from build123d import *

# Parameters (mm, degrees)
BLANKSKE_W           = 127
BLANKSKE_H           = 43.18
BLANK_DEPTH          = 25.4
TOOTHCUTSIM_DEPTH    = 137.523523248
TEETHCUTS_COUNT      = 9
TEETHCUTS_PITCH      = 15.959290662
BOSS_EXTRUDE1_DEPTH  = 25.4
MIRROR1_COPY_1_DEPTH = 137.523523248
MIRROR1_COPY_2_DEPTH = 137.523523248
MIRROR1_COPY_3_DEPTH = 137.523523248
MIRROR1_COPY_4_DEPTH = 137.523523248
MIRROR1_COPY_5_DEPTH = 137.523523248
MIRROR1_COPY_6_DEPTH = 137.523523248
MIRROR1_COPY_7_DEPTH = 137.523523248
MIRROR1_COPY_8_DEPTH = 137.523523248
CUT_EXTRUDE1_DEPTH   = 232.151804304
SKETCH5_W            = 249.809436719
SKETCH5_H            = 19.05
CUT_EXTRUDE2_DEPTH   = 232.151804304
BOSS_EXTRUDE2_DEPTH  = 6.35


with BuildPart() as part:
    # BlankSke → Blank (new body)
    with BuildSketch(Plane.XY):
        with Locations((63.5, 21.59)):
            Rectangle(BLANKSKE_W, BLANKSKE_H)
    blank = extrude(amount=-BLANK_DEPTH)

    # TooCutSkeSim → ToothCutSim (cut, through all)
    with BuildSketch(Plane.XY):
        Polygon((2.250111678, 31.75), (-2.250111678, 31.75), (-6.4195363, 43.2054), (6.4195363, 43.2054), align=None)
    toothcutsim = extrude(amount=-TOOTHCUTSIM_DEPTH, mode=Mode.SUBTRACT)

    # TeethCuts: ToothCutSim ×9
    with Locations(*[(i * TEETHCUTS_PITCH, 0, 0) for i in range(1, TEETHCUTS_COUNT)]):
        add(toothcutsim, mode=Mode.SUBTRACT)

    # Sketch3 → Boss-Extrude1 (add)
    with BuildSketch(Plane(origin=(0, 0, -25.4), x_dir=(-1, 0, 0), z_dir=(0, 0, -1))):
        with BuildLine():
            Line((-127.960169835, 127), (-5.150733116, 127))
            ThreePointArc((-5.150733116, 127), (58.349266884, 63.5), (-5.150733116, 0))
            Line((-5.150733116, 0), (-127.960169835, 0))
            ThreePointArc((-127.960169835, 0), (-191.460169835, 63.5), (-127.960169835, 127))
        make_face()
        with BuildLine():
            Line((-127.960169835, 95.25), (-5.150733116, 95.25))
            ThreePointArc((-5.150733116, 95.25), (26.599266884, 63.5), (-5.150733116, 31.75))
            Line((-5.150733116, 31.75), (-127.960169835, 31.75))
            ThreePointArc((-127.960169835, 31.75), (-159.710169835, 63.5), (-127.960169835, 95.25))
        make_face(mode=Mode.SUBTRACT)
    extrude(amount=-BOSS_EXTRUDE1_DEPTH)

    # Mirror1: Blank, ToothCutSim across plane
    add(blank.mirror(Plane.ZX.offset(63.5)))
    add(toothcutsim.mirror(Plane.ZX.offset(63.5)), mode=Mode.SUBTRACT)

    # Mirror1 copy 1 sketch → Mirror1 copy 1 (cut, through all)
    with BuildSketch(Plane(origin=(15.959290662, 127, 0), x_dir=(1, 0, 0), z_dir=(0, 0, 1))):
        Polygon((2.250111678, -31.75), (-2.250111678, -31.75), (-6.4195363, -43.2054), (6.4195363, -43.2054), align=None)
    extrude(amount=-MIRROR1_COPY_1_DEPTH, mode=Mode.SUBTRACT)

    # Mirror1 copy 2 sketch → Mirror1 copy 2 (cut, through all)
    with BuildSketch(Plane(origin=(31.918581324, 127, 0), x_dir=(1, 0, 0), z_dir=(0, 0, 1))):
        Polygon((2.250111678, -31.75), (-2.250111678, -31.75), (-6.4195363, -43.2054), (6.4195363, -43.2054), align=None)
    extrude(amount=-MIRROR1_COPY_2_DEPTH, mode=Mode.SUBTRACT)

    # Mirror1 copy 3 sketch → Mirror1 copy 3 (cut, through all)
    with BuildSketch(Plane(origin=(47.877871986, 127, 0), x_dir=(1, 0, 0), z_dir=(0, 0, 1))):
        Polygon((2.250111678, -31.75), (-2.250111678, -31.75), (-6.4195363, -43.2054), (6.4195363, -43.2054), align=None)
    extrude(amount=-MIRROR1_COPY_3_DEPTH, mode=Mode.SUBTRACT)

    # Mirror1 copy 4 sketch → Mirror1 copy 4 (cut, through all)
    with BuildSketch(Plane(origin=(63.837162648, 127, 0), x_dir=(1, 0, 0), z_dir=(0, 0, 1))):
        Polygon((2.250111678, -31.75), (-2.250111678, -31.75), (-6.4195363, -43.2054), (6.4195363, -43.2054), align=None)
    extrude(amount=-MIRROR1_COPY_4_DEPTH, mode=Mode.SUBTRACT)

    # Mirror1 copy 5 sketch → Mirror1 copy 5 (cut, through all)
    with BuildSketch(Plane(origin=(79.79645331, 127, 0), x_dir=(1, 0, 0), z_dir=(0, 0, 1))):
        Polygon((2.250111678, -31.75), (-2.250111678, -31.75), (-6.4195363, -43.2054), (6.4195363, -43.2054), align=None)
    extrude(amount=-MIRROR1_COPY_5_DEPTH, mode=Mode.SUBTRACT)

    # Mirror1 copy 6 sketch → Mirror1 copy 6 (cut, through all)
    with BuildSketch(Plane(origin=(95.755743972, 127, 0), x_dir=(1, 0, 0), z_dir=(0, 0, 1))):
        Polygon((2.250111678, -31.75), (-2.250111678, -31.75), (-6.4195363, -43.2054), (6.4195363, -43.2054), align=None)
    extrude(amount=-MIRROR1_COPY_6_DEPTH, mode=Mode.SUBTRACT)

    # Mirror1 copy 7 sketch → Mirror1 copy 7 (cut, through all)
    with BuildSketch(Plane(origin=(111.715034634, 127, 0), x_dir=(1, 0, 0), z_dir=(0, 0, 1))):
        Polygon((2.250111678, -31.75), (-2.250111678, -31.75), (-6.4195363, -43.2054), (6.4195363, -43.2054), align=None)
    extrude(amount=-MIRROR1_COPY_7_DEPTH, mode=Mode.SUBTRACT)

    # Mirror1 copy 8 sketch → Mirror1 copy 8 (cut, through all)
    with BuildSketch(Plane(origin=(127.674325296, 127, 0), x_dir=(1, 0, 0), z_dir=(0, 0, 1))):
        Polygon((2.250111678, -31.75), (-2.250111678, -31.75), (-6.4195363, -43.2054), (6.4195363, -43.2054), align=None)
    extrude(amount=-MIRROR1_COPY_8_DEPTH, mode=Mode.SUBTRACT)

    # Sketch4 → Cut-Extrude1 (cut, through all)
    with BuildSketch(Plane(origin=(0, 0, -25.4), x_dir=(-1, 0, 0), z_dir=(0, 0, -1))):
        with BuildLine():
            Line((4.314647241, 9.525), (-124.523078394, 9.525))
            ThreePointArc((-124.523078394, 9.525), (-127.698078394, 12.7), (-124.523078394, 15.875))
            Line((-124.523078394, 15.875), (4.314647241, 15.875))
            ThreePointArc((4.314647241, 15.875), (7.489647241, 12.7), (4.314647241, 9.525))
        make_face()
        with BuildLine():
            Line((0, 111.125), (-124.523078394, 111.125))
            ThreePointArc((-124.523078394, 111.125), (-127.698078394, 114.3), (-124.523078394, 117.475))
            Line((-124.523078394, 117.475), (0, 117.475))
            ThreePointArc((0, 117.475), (3.175, 114.3), (0, 111.125))
        make_face()
    extrude(amount=-CUT_EXTRUDE1_DEPTH, mode=Mode.SUBTRACT)

    # Sketch5 → Cut-Extrude2 (cut, through all)
    with BuildSketch(Plane(origin=(0, 0, 0), x_dir=(1, 0, 0), z_dir=(0, 1, 0))):
        with Locations((66.555451476, 9.525)):
            Rectangle(SKETCH5_W, SKETCH5_H)
    extrude(amount=CUT_EXTRUDE2_DEPTH, mode=Mode.SUBTRACT)

    # Sketch6 → Boss-Extrude2 (add)
    with BuildSketch(Plane(origin=(0, 0, -25.4), x_dir=(-1, 0, 0), z_dir=(0, 0, -1))):
        Polygon((-191.364398064, 117.861523458), (-191.364398064, 143.261523458), (58.349266884, 143.261523458), (58.349266884, 117.861523458), (58.349266884, 63.5), (13.664264486, 117.861523458), (-144.531259298, 117.861523458), (-191.364398064, 66.98623618), align=None)
    extrude(amount=-BOSS_EXTRUDE2_DEPTH)


solid = part.part
Work out the finished part from the listing and answer in its coordinate system (mm). Give positions to 0.01 mm unless a question says otherwise; leave off trailing zeros. Write each loop counter-clockwise with the first axis right and the second up, starting at its lowest first coordinate (ties: lowest second). Pieces come first, ordered by that corner, then holes.
Q1. For a pull along X with two mould halves and no side action, classify faces 1 (the face through (-41.982, 20.947, -22.269)), 2 (the face through (100.1, 37.5, -22.2)) as released by +X, released by -X, zero draft, split by the parting line, or undercut.
Answer:
face 1: released by -X
face 2: undercut
Q2. The part is cut by section C-C on y = 49. Give the vertices of the cut face in (x, z).
Answer:
outline: (-56.67, -25.4) - (-23.09, -25.4) - (-23.09, -19.05) - (-56.67, -19.05) - close; (156.21, -25.4) - (189.78, -25.4) - (189.78, -19.05) - (156.21, -19.05) - close
Q3. The part is cut by section D-D on x = -41. Give the vertices of the cut face in (y, z).
Answer:
outline: (19.88, -25.4) - (143.26, -25.4) - (143.26, -19.05) - (19.88, -19.05) - close
Q4. The part is cut by section B-B on z = -22.5. State how many separate pieces and enclosed holes the cut face has, and give its area (3 significant figures).
Answer:
separate pieces: 1
enclosed holes: 3
area: 22,700 mm2
Q5. Straight lines are drawn through the part: L1, parallel to Y at x = 33.5, z = -21.5 (3 decimals); L2, parallel to Y at x = 6.5, z = -20 (3 decimals); L3, parallel to Y at x = -6.5, z = -24. For each, find the intervals that lie inside material, in ascending order.
Answer:
L1: y = 0 to 9.525, 15.875 to 31.75, 95.25 to 111.125, 117.475 to 143.262
L2: y = 0 to 9.525, 15.875 to 43.18, 83.82 to 111.125, 117.475 to 143.262
L3: y = 1.08 to 10.4, 15 to 33.96, 93.04 to 143.26
Q6. The part is cut by section A-A on y = 114.3. Give the vertices of the cut face in (x, z) (3 decimals).
Answer:
outline: (-58.349, -25.4) - (-3.175, -25.4) - (-3.175, -19.05) - (-58.349, -19.05) - close; (127.698, -25.4) - (191.364, -25.4) - (191.364, -19.05) - (127.698, -19.05) - close
